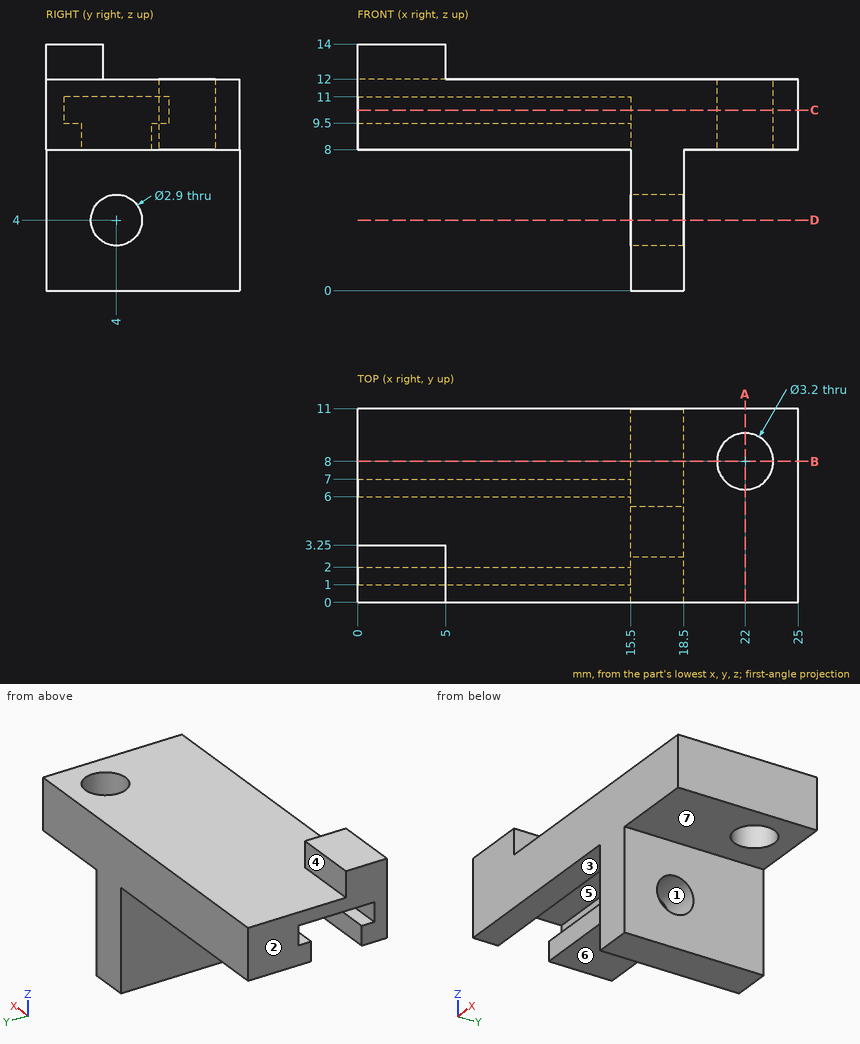
Input: dimensioned drawing with shaded views. Units: mm. Origin: part minimum x, y, z. A direction names the side the tool comes from. Coordinates: 2 decimals unless noted, no trailing zeros. Order: outer loops, then holes, each group sorted by start corner. A loop starts at its lowest first (then second) coordinate and runs counter-clockwise, first axis right, second up. Notation, with made-up numbers: (13.25, -20) -> (22.25, -20) arc R17 cw to (22.25, -4) -> close; hole circle Ø1 at (80, 59). An arc over 180 degrees is marked (long way). Use CSV: the item, a comma, the result in double quotes.
1) Section A-A on x = 22. Output: boundary loops of the cut face in (y, z), then the cut area to 3 significant figures.
Findings:
outline,"(0, 8) -> (6.4, 8) -> (6.4, 12) -> (0, 12) -> close; (9.6, 8) -> (11, 8) -> (11, 12) -> (9.6, 12) -> close"
area,"31.2 mm^2"
2) Section C-C on z = 10.25. Output: boundary loops of the cut face in (x, y).
Findings:
outline,"(0, 0) -> (25, 0) -> (25, 11) -> (0, 11) -> (0, 7) -> (15.5, 7) -> (15.5, 1) -> (0, 1) -> close; hole circle Ø3.2 at (22, 8)"
3) Line query: line 1 (Z direction, x = 10.5, y = 6.5); line 2 (Y direction, x = 10.5, z = 8.25); line 3 (Z direction, x = 17.25, y = 4). Output: solid intervals per line, ascending.
Findings:
line 1,"z = 8 to 9.5, 11 to 12"
line 2,"y = 0 to 2, 6 to 11"
line 3,"z = 0 to 2.55, 5.45 to 12"
4) Mould query, pull axis Z, two halves, no side actions, for the marked faces 1, 2 and 3. Classes: +Z half, -Z half, draft (parallel to the pull), parting line (faces both ways), or undercut.
Findings:
face 1,"undercut"
face 2,"draft"
face 3,"-Z half"
5) Section B-B on y = 8. Output: boundary loops of the cut face in (x, z), then the cut area to 3 significant figures.
Findings:
outline,"(0, 8) -> (15.5, 8) -> (15.5, 0) -> (18.5, 0) -> (18.5, 8) -> (20.4, 8) -> (20.4, 12) -> (0, 12) -> close; (23.6, 8) -> (25, 8) -> (25, 12) -> (23.6, 12) -> close"
area,"111 mm^2"
6) Section D-D on z = 4. Output: boundary loops of the cut face in (x, y).
Findings:
outline,"(15.5, 0) -> (18.5, 0) -> (18.5, 2.55) -> (15.5, 2.55) -> close; (15.5, 5.45) -> (18.5, 5.45) -> (18.5, 11) -> (15.5, 11) -> close"
7) Access query for the marked faces 4, 5, 6 and 7. Directions: +Z, -Z, +X, -X, +Y, -Y. A direction counts if a zero-diameter tool reaches every point of the face in a straight line with its end or side. Return the directions, or none.
Findings:
face 4,"+Z, +X, -X, +Y"
face 5,"-X"
face 6,"-Z, -X, +Y, -Y"
face 7,"-Z, +X, +Y, -Y"
8) Pin query (flat end, axial travel): pin 1 Ø6 at (x, y) = (9, 6) entering from +Z; pin 2 Ø6.5 at (y, z) = (5, 2) entering from +X; pin 3 Ø4 at (x, y) = (11.5, 8.5) entering from -Z. Return the tip coordinate at first contact, or that it passes through.
Findings:
pin 1,"stops at z = 12"
pin 2,"stops at x = 18.5"
pin 3,"stops at z = 8"
